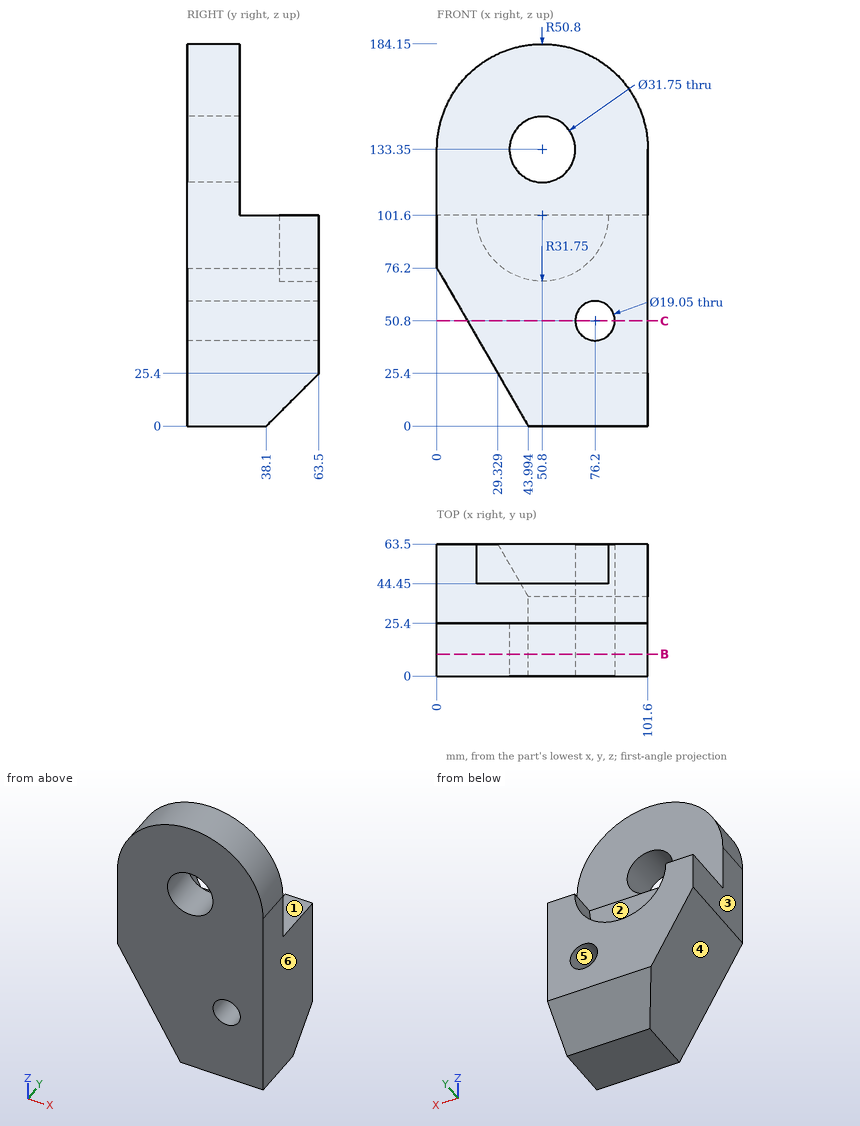
Could you check a few things on this drawing? It's one solid part, dimensions in mm from its lowest x, y, z. A direction names the side the tool comes from. Coordinates: 2 decimals unless noted, no trailing zeros. Write each loop counter-clockwise with the first axis right and the second up, starting at its lowest first coordinate (ties: lowest second). Pieces come first, ordered by that corner, then holes. Notation, with made-up numbers: (29, -7.5) - (77, -7.5) arc R21 ccw to (77, 23.5) - close; hole circle Ø2 at (33.25, 29). An arc over 180 degrees is marked (long way). Write item = value, one per line.
1) Please list where these lines run through material, in increasing order: line 1 (X direction, y = 14.25, z = 133.35) (1 decimal); line 2 (Z direction, x = 50, y = 17) (1 decimal); line 3 (Z direction, x = 76.2, y = 35.5) (1 decimal). Write a range as [from, to].
Result set:
line_1 = [0, 34.9], [66.7, 101.6]
line_2 = [0, 117.5], [149.2, 184.1]
line_3 = [0, 41.3], [60.3, 101.6]
2) Suppose I cut it at C-C on z = 50.8. Please give me the cut outline in (x, y) (1 decimal).
Result set:
outline = (14.7, 0) - (66.7, 0) - (66.7, 63.5) - (14.7, 63.5) - close; (85.7, 0) - (101.6, 0) - (101.6, 63.5) - (85.7, 63.5) - close
3) Suppose I cut it at B-B on y = 10.5. State how many separate pieces and enclosed holes the cut face has, plus the area to 3 significant figures.
Result set:
separate_pieces = 1
enclosed_holes = 2
area = 14,800 mm2
4) For the marked faces 1, 2 and 3, which set-ups out of +Z, -Z, +X, -X, +Y, -Y let a thin tool reach every point of the face, with its end or its side?
Result set:
face_1 = +Z, +X, -X, +Y
face_2 = +Z, +Y
face_3 = +Z, -Z, -X, +Y, -Y
5) We'd pull the mould along Z, two halves only. Please class the marked faces 4, 5 and 6: +Z half, -Z half, draft (parallel to the pull), parting line (faces both ways), or undercut.
Result set:
face_4 = -Z half
face_5 = undercut
face_6 = draft
6) Will these pins go through, and if not, where does the flat tip stop? pin 1 Ø9.5 at (x, z) = (54, 83) entering from +Y; pin 2 Ø12 at (x, z) = (42, 138.5) entering from +Y; pin 3 Ø25 at (x, z) = (76.2, 50.8) entering from -Y; pin 4 Ø1 at (x, y) = (16.5, 30.5) entering from -Z (1 decimal).
Result set:
pin_1 = 44.45
pin_2 = 25.4
pin_3 = 0
pin_4 = 46.8
